Verification items for this drawing (mm, ordinates from the low corner). Round coordinates to 2 decimals unless told otherwise and drop trailing zeros. Loops run counter-clockwise (first coordinate to the right, second up) from the corner with the lowest first, then second, coordinate; pieces in that order, holes last. Notation, with made-up numbers: (31.25, 1) -> (63.25, 1) arc R33 cw to (63.25, 32) -> close; hole circle Ø2 at (27.25, 29.5). An arc over 180 degrees is marked (long way). One line per question, with ' | ' between items.
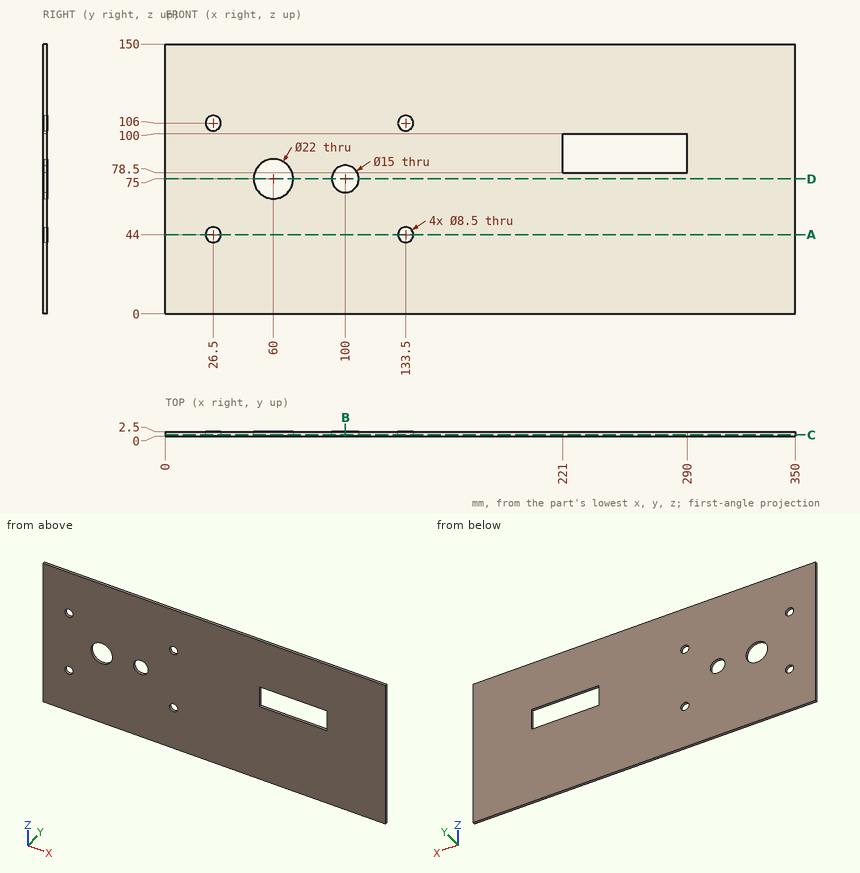
(1) Scan lines: probe 1 along Z at (x, y) = (133.5, 1.35); probe 2 along Z at (x, y) = (277.5, 2.2); probe 3 along X at (y, z) = (1.4, 79). Record each from-to range of solid material in increasing order.
Answer:
probe 1: z = 0 to 39.75, 48.25 to 101.75, 110.25 to 150 | probe 2: z = 0 to 78.5, 100 to 150 | probe 3: x = 0 to 49.75, 70.25 to 93.66, 106.34 to 221, 290 to 350
(2) Sectioned sample at C-C, the plane y = 0.8. Record the cut outline in (x, z), and give its area (3 significant figures).
Answer:
outline: (0, 0) -> (350, 0) -> (350, 150) -> (0, 150) -> close; hole circle Ø8.5 at (26.5, 44); hole circle Ø8.5 at (26.5, 106); hole circle Ø22 at (60, 75); hole circle Ø15 at (100, 75); hole circle Ø8.5 at (133.5, 44); hole circle Ø8.5 at (133.5, 106); hole (221, 78.5) -> (290, 78.5) -> (290, 100) -> (221, 100) -> close | area: 50,200 mm2
(3) Sectioned sample at B-B, the plane x = 100. Record the cut outline in (y, z).
Answer:
outline: (0, 0) -> (2.5, 0) -> (2.5, 67.5) -> (0, 67.5) -> close; (0, 82.5) -> (2.5, 82.5) -> (2.5, 150) -> (0, 150) -> close
(4) Sectioned sample at D-D, the plane z = 75. Record the cut outline in (x, y), and give its area (4 significant figures).
Answer:
outline: (0, 0) -> (49, 0) -> (49, 2.5) -> (0, 2.5) -> close; (71, 0) -> (92.5, 0) -> (92.5, 2.5) -> (71, 2.5) -> close; (107.5, 0) -> (350, 0) -> (350, 2.5) -> (107.5, 2.5) -> close | area: 782.5 mm2
(5) Sectioned sample at A-A, the plane z = 44. Record the cut outline in (x, y).
Answer:
outline: (0, 0) -> (22.25, 0) -> (22.25, 2.5) -> (0, 2.5) -> close; (30.75, 0) -> (129.25, 0) -> (129.25, 2.5) -> (30.75, 2.5) -> close; (137.75, 0) -> (350, 0) -> (350, 2.5) -> (137.75, 2.5) -> close
